from build123d import *

# Parameters (mm, degrees)
SKETCH1_W                  = 8.5
SKETCH1_H                  = 8.5
BOSS_EXTRUDE1_DEPTH        = 56.75
BOSS_EXTRUDE1_DEPTH_BACK   = 56.75
BOSS_EXTRUDE1_2_DEPTH      = 56.75
BOSS_EXTRUDE1_2_DEPTH_BACK = 56.75
BOSS_EXTRUDE1_3_DEPTH      = 56.75
BOSS_EXTRUDE1_3_DEPTH_BACK = 56.75
BOSS_EXTRUDE1_4_DEPTH      = 56.75
BOSS_EXTRUDE1_4_DEPTH_BACK = 56.75
SKETCH2_W                  = 100
SKETCH2_H                  = 100
BOSS_EXTRUDE2_DEPTH        = 50.25
BOSS_EXTRUDE2_DEPTH_BACK   = 50.25
CHAMFER2_SIZE              = 1
FILLET1_R                  = 1
BOSS_EXTRUDE3_DEPTH        = 6


with BuildPart() as part:
    # Sketch1 → Boss-Extrude1 (new body, two sides)
    with BuildSketch(Plane.XY) as boss_extrude1_sk:
        with Locations((-45.75, 45.75)):
            Rectangle(SKETCH1_W, SKETCH1_H)
    extrude(amount=BOSS_EXTRUDE1_DEPTH)
    extrude(boss_extrude1_sk.sketch, amount=-BOSS_EXTRUDE1_DEPTH_BACK)



with BuildPart() as body_2:
    # Sketch1 → Boss-Extrude1 2 (new body, two sides)
    with BuildSketch(Plane.XY) as boss_extrude1_2_sk:
        with Locations((45.75, 45.75)):
            Rectangle(SKETCH1_W, SKETCH1_H)
    extrude(amount=BOSS_EXTRUDE1_2_DEPTH)
    extrude(boss_extrude1_2_sk.sketch, amount=-BOSS_EXTRUDE1_2_DEPTH_BACK)


with BuildPart() as body_3:
    # Sketch1 → Boss-Extrude1 3 (new body, two sides)
    with BuildSketch(Plane.XY) as boss_extrude1_3_sk:
        with Locations((45.75, -45.75)):
            Rectangle(SKETCH1_W, SKETCH1_H)
    extrude(amount=BOSS_EXTRUDE1_3_DEPTH)
    extrude(boss_extrude1_3_sk.sketch, amount=-BOSS_EXTRUDE1_3_DEPTH_BACK)


with BuildPart() as body_4:
    # Sketch1 → Boss-Extrude1 4 (new body, two sides)
    with BuildSketch(Plane.XY) as boss_extrude1_4_sk:
        with Locations((-45.75, -45.75)):
            Rectangle(SKETCH1_W, SKETCH1_H)
    extrude(amount=BOSS_EXTRUDE1_4_DEPTH)
    extrude(boss_extrude1_4_sk.sketch, amount=-BOSS_EXTRUDE1_4_DEPTH_BACK)


with BuildPart() as part_1:
    add(part.part)

    add(body_2.part)  # Boss-Extrude2 merges body 2

    add(body_3.part)  # Boss-Extrude2 merges body 3

    add(body_4.part)  # Boss-Extrude2 merges body 4
    # Sketch2 → Boss-Extrude2 (add, two sides)
    with BuildSketch(Plane.XY) as boss_extrude2_sk:
        Rectangle(SKETCH2_W, SKETCH2_H)
    extrude(amount=BOSS_EXTRUDE2_DEPTH)
    extrude(boss_extrude2_sk.sketch, amount=-BOSS_EXTRUDE2_DEPTH_BACK)

    # Chamfer2
    chamfer2_edges = [part_1.edges().sort_by_distance(p)[0] for p in [
        (50, 45.75, 56.75),
        (41.5, 45.75, -56.75),
        (45.75, 50, 56.75),
        (41.5, 45.75, 56.75),
        (45.75, 41.5, 56.75),
        (45.75, 41.5, -56.75),
        (-50, -45.75, -56.75),
        (-45.75, -41.5, -56.75),
        (-41.5, -45.75, -56.75),
        (50, 45.75, -56.75),
        (-45.75, -50, -56.75),
        (-50, -45.75, 56.75),
        (-45.75, -50, 56.75),
        (-41.5, -45.75, 56.75),
        (-45.75, -41.5, 56.75),
        (-50, 45.75, -56.75),
        (-45.75, 50, -56.75),
        (-41.5, 45.75, -56.75),
        (-45.75, 41.5, -56.75),
        (-50, 45.75, 56.75),
        (-45.75, 41.5, 56.75),
        (-41.5, 45.75, 56.75),
        (-45.75, 50, 56.75),
        (50, -45.75, -56.75),
        (45.75, -50, -56.75),
        (41.5, -45.75, -56.75),
        (45.75, -41.5, -56.75),
        (50, -45.75, 56.75),
        (45.75, -41.5, 56.75),
        (41.5, -45.75, 56.75),
        (45.75, -50, 56.75),
        (45.75, 50, -56.75),
    ]]
    chamfer(chamfer2_edges, length=CHAMFER2_SIZE)

    # Fillet1
    fillet1_edges = [part_1.edges().sort_by_distance(p)[0] for p in [
        (50, -50, 0),
        (-50, -50, 0),
        (-50, 50, 0),
        (50, 50, 0),
    ]]
    fillet(fillet1_edges, radius=FILLET1_R)

    # Sketch3 → Boss-Extrude3 (add)
    with BuildSketch(Plane.XY.offset(50.25)):
        Polygon((-41.5, 50), (41.5, 50), (41.5, 41.5), (50, 41.5), (50, -41.5), (41.5, -41.5), (41.5, -50), (-41.5, -50), (-41.5, -41.5), (-50, -41.5), (-50, 41.5), (-41.5, 41.5), align=None)
    boss_extrude3 = extrude(amount=BOSS_EXTRUDE3_DEPTH)

    # Mirror1: Boss-Extrude3 across plane
    add(boss_extrude3.mirror(Plane.XY))


solid = part_1.part
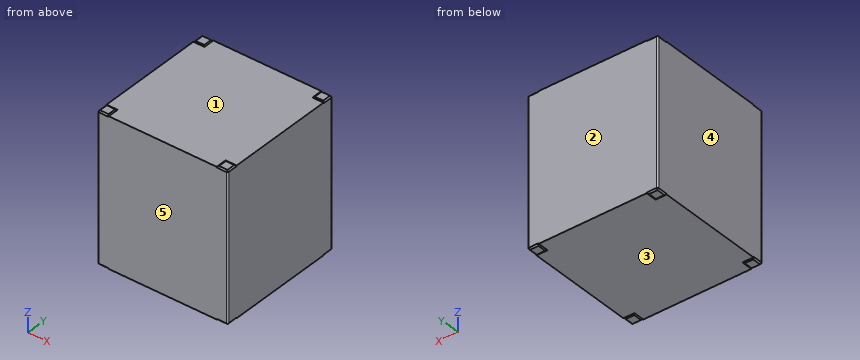
Input: part model. Units: mm. Frame: model coordinates. Face numbers are marked on the shaded views. A direction names the side the tool comes from. Give positions to 0.01 mm unless a question says otherwise; leave off trailing zeros. Write item = value, one per line. Start each with the question number.
1) Reachability of the marked faces 1 and 2 from +Z, -Z, +X, -X, +Y, -Y: full face, straight path, thin tool, end or side. Return the list, or none.
2) First-contact query: pin 1 Ø8 at (x, y) = (30, -26) entering from +Z; pin 2 Ø0.6 at (x, z) = (-46.5, 56) entering from -Y. Flat tips, straight axial feed; report the tip coordinate or a pass-through.
3) Material intervals for line 1 along Z through (x, y) = (26, -6), sorted ascending. Write a range as [from, to].
4) Draft query along Y for the marked faces 3, 4 and 5. Return one class per face: +Y half, -Y half, draft (parallel to the pull), parting line (faces both ways), or undercut.
Solved:
q1.face_1 = +Z
q1.face_2 = +Z, -Z, +X, -X, +Y
q2.pin_1 = 56.25
q2.pin_2 = -50
q3.line_1 = [-56.25, 56.25]
q4.face_3 = undercut
q4.face_4 = draft
q4.face_5 = -Y half
